Can you work these out from the model? Positions are in its coordinate system, mm. A direction names the side the tool comes from. Coordinates: 2 decimals unless noted, no trailing zeros. Order: outer loops, then holes, each group sorted by start corner. A loop starts at its lowest first (then second) coordinate and runs counter-clockwise, first axis right, second up. Notation, with made-up numbers: (67.5, 17.5) - (73.5, 17.5) arc R21 cw to (73.5, 43.5) - close; hole circle Ø6 at (81.5, 0). An arc over 180 degrees is marked (long way). Use a Markdown table: item, result. Add a question column.
(1) I want a section at A-A (y = 14). List the corners of the cut face in (x, z) for me, and give its area (3 significant figures).
(2) For pin 1 Ø1 at (x, y) = (22.5, -33.5) entering from +Z, with a flat end and sliding along its axis, tell me the tip position at first contact or that it passes through.
(3) If I drill on L1, parallel to X at y = -18.5, z = 3.05; L2, parallel to X at y = -12, z = 4.7; L3, parallel to X at y = -4, z = 3.2, over which ranges is the centre line in solid material (lowest first)? Write a range as [from, to].
(4) On a 3-axis mill with a long thin cutter (end or side, diameter ignored), from which of +Z, -Z, +X, -X, +Y, -Y can I reach the whole of each face in a straight line? I mean faces 5 (the cylindrical face through (3.409, 36.106, 3.521)), 6 (the flat face through (20, -21, 2)), 7 (the flat face through (-25, -20, 2)). Say none if no direction works.
(5) I want a section at C-C (x = 16.5). List the corners of the cut face in (y, z) for me.
(6) I want a section at B-B (z = 1). List the corners of the cut face in (x, y) for me.
(7) We'd pull the mould along Y, two halves only. Please class faces 1 (the flat face through (22, -62.075, 2)), 2 (the flat face through (-20.5, -11.8, 0)), 3 (the flat face through (-23, -53, 2)), 4 (the cylindrical face through (-23.237, -27.823, 3.521)): pulls with the +Y half, pulls with the -Y half, needs draft (parallel to the pull), parting line crosses it, or undercut.
```python
from build123d import *

# Parameters (mm, degrees)
F1_DEPTH = 5
F2_R     = 1
F3_DEPTH = 3
F4_R     = 8


with BuildPart() as f1:
    # F0 (on Top) → F1 (new body)
    with BuildSketch(Plane.XY):
        with BuildLine():
            ThreePointArc((25, 22.501486), (0, 37.925084), (-25, 22.501486))
            Line((-25, 22.501486), (-25, -62.074916))
            Line((-25, -62.074916), (-20, -62.074916))
            Line((-20, -62.074916), (-20, 21.255084))
            ThreePointArc((-20, 21.255084), (0, 32.925084), (20, 21.255084))
            Line((20, 21.255084), (20, -62.074916))
            Line((20, -62.074916), (25, -62.074916))
            Line((25, -62.074916), (25, 22.501486))
        make_face()
    extrude(amount=F1_DEPTH)

    # F2 (on face) → F3 (cut)
    with BuildSketch(Plane.XY.offset(5)):
        with Locations((-22.5, -13.498514)):
            Circle(F2_R)
        with Locations((-22.5, -8.498514)):
            Circle(F2_R)
        with Locations((-22.5, -3.498514)):
            Circle(F2_R)
        with Locations((-22.5, 1.501486)):
            Circle(F2_R)
        with Locations((-22.5, 6.501486)):
            Circle(F2_R)
        with Locations((-22.5, 11.501486)):
            Circle(F2_R)
        with Locations((-22.5, 16.501486)):
            Circle(F2_R)
        with Locations((-22.5, 21.501486)):
            Circle(F2_R)
        with Locations((-19.943857, 25.79871)):
            Circle(F2_R)
        with Locations((-16.464199, 29.38925)):
            Circle(F2_R)
        with Locations((-12.350201, 32.230908)):
            Circle(F2_R)
        with Locations((-7.760369, 34.214201)):
            Circle(F2_R)
        with Locations((-2.871543, 35.262714)):
            Circle(F2_R)
        with Locations((2.871543, 35.262714)):
            Circle(F2_R)
        with Locations((7.760369, 34.214201)):
            Circle(F2_R)
        with Locations((12.350201, 32.230908)):
            Circle(F2_R)
        with Locations((16.464199, 29.38925)):
            Circle(F2_R)
        with Locations((19.943857, 25.79871)):
            Circle(F2_R)
        with Locations((22.5, 21.501486)):
            Circle(F2_R)
        with Locations((22.5, 16.501486)):
            Circle(F2_R)
        with Locations((22.5, 11.501486)):
            Circle(F2_R)
        with Locations((22.5, 6.501486)):
            Circle(F2_R)
        with Locations((22.5, 1.501486)):
            Circle(F2_R)
        with Locations((22.5, -3.498514)):
            Circle(F2_R)
        with Locations((22.5, -8.498514)):
            Circle(F2_R)
        with Locations((22.5, -13.498514)):
            Circle(F2_R)
        with Locations((22.5, -18.498514)):
            Circle(F2_R)
        with Locations((22.5, -23.498514)):
            Circle(F2_R)
        with Locations((22.5, -28.498514)):
            Circle(F2_R)
        with Locations((22.5, -33.498514)):
            Circle(F2_R)
        with Locations((22.5, -48.498514)):
            Circle(F2_R)
        with Locations((22.5, -38.498514)):
            Circle(F2_R)
        with Locations((22.5, -43.498514)):
            Circle(F2_R)
        with Locations((22.5, -53.498514)):
            Circle(F2_R)
        with Locations((-22.5, -18.498514)):
            Circle(F2_R)
        with Locations((-22.5, -23.498514)):
            Circle(F2_R)
        with Locations((-22.5, -28.498514)):
            Circle(F2_R)
        with Locations((-22.5, -33.498514)):
            Circle(F2_R)
        with Locations((-22.5, -38.498514)):
            Circle(F2_R)
        with Locations((-22.5, -43.498514)):
            Circle(F2_R)
        with Locations((-22.5, -48.498514)):
            Circle(F2_R)
        with Locations((-22.5, -53.498514)):
            Circle(F2_R)
        with Locations((-22.5, -58.498514)):
            Circle(F2_R)
        with Locations((22.5, -58.498514)):
            Circle(F2_R)
    extrude(amount=-F3_DEPTH, mode=Mode.SUBTRACT)

    # F4
    f4_edges = [f1.edges().sort_by_distance(p)[0] for p in [
        (-25, 22.501486, 2.5),
        (-20, 21.255084, 2.5),
        (25, 22.501486, 2.5),
        (20, 21.255084, 2.5),
    ]]
    fillet(f4_edges, radius=F4_R)


solid = f1.part
```
Answers follow:
| question | item | result |
|---|---|---|
| 1 | outline | (-25, 0) - (-20, 0) - (-20, 5) - (-25, 5) - close; (20, 0) - (25, 0) - (25, 5) - (20, 5) - close |
| 1 | area | 50.0 mm² |
| 2 | pin 1 | stops at z = 2 |
| 3 | L1 | x = [-25, -23.5], [-21.5, -20], [20, 21.5], [23.5, 25] |
| 3 | L2 | x = [-25, -20], [20, 25] |
| 3 | L3 | x = [-25, -23.37], [-21.63, -20], [20, 21.63], [23.37, 25] |
| 4 | face 5 | +Z |
| 4 | face 6 | +Z, -Z, -Y |
| 4 | face 7 | +Z, -Z, -X, +Y, -Y |
| 5 | outline | (25.94, 0) - (32.54, 0) - (32.54, 5) - (30.39, 5) - (30.39, 2) - (28.39, 2) - (28.39, 5) - (25.94, 5) - close |
| 6 | outline | (-25, -62.07) - (-20, -62.07) - (-20, 18.91) arc R8 cw to (-18.41, 23.69) arc R22.97 cw to (18.41, 23.69) arc R8 cw to (20, 18.91) - (20, -62.07) - (25, -62.07) - (25, 20.44) arc R8 ccw to (23.81, 24.64) arc R27.97 ccw to (-23.81, 24.64) arc R8 ccw to (-25, 20.44) - close |
| 7 | face 1 | pulls with the -Y half |
| 7 | face 2 | needs draft |
| 7 | face 3 | undercut |
| 7 | face 4 | undercut |
